Here's how the part is built. I have some questions about the finished solid (model axes, mm). A direction names the side the tool comes from. Coordinates: 2 decimals unless noted, no trailing zeros. Write each loop counter-clockwise with the first axis right and the second up, starting at its lowest first coordinate (ties: lowest second). Pieces come first, ordered by that corner, then holes. Notation, with made-up numbers: (49, -24) -> (83, -24) arc R8 cw to (83, -9) -> close; hole circle Ø5 at (-0.5, 25). An arc over 180 degrees is marked (long way). Use a Markdown table: item, result. Add a question column.
Item 1: If we mould it in two halves opening along Z, with no side actions, what happens to faces 6 (the flat face through (-2.2, 23, 0)), 7 (the flat face through (0, -34.6, 0)), 8 (the flat face through (-2.2, -2, 0)), 9 (the cylindrical face through (1.08, 9.86, 4.88))? For each: pulls with the +Z half, pulls with the -Z half, needs draft (parallel to the pull), parting line crosses it, or undercut.
Item 2: On a 3-axis mill with a long thin cutter (end or side, diameter ignored), from which of +Z, -Z, +X, -X, +Y, -Y can I reach the whole of each face in a straight line? I mean faces 1 (the flat face through (0, 91, 0)), 2 (the cylindrical face through (3.695, -17.058, 1.532)), 3 (the flat face through (-3, 20, 0)), 4 (the cylindrical face through (3.695, 55.003, -1.532)), 5 (the flat face through (-2.2, 72, 0)). Say none if no direction works.
Item 3: Imagine slicing it at D-D, the plane y = 6. Write out the boundary of the cut face in (x, z), and give its area (3 significant figures).
Item 4: Will these pins go through, and if not, where does the flat tip stop? pin 1 Ø0.8 at (x, y) = (-3, -3.5) entering from -Z; pin 2 Ø1.7 at (x, y) = (-3, 71.5) entering from -Z; pin 3 Ø1.7 at (x, y) = (-2.5, 71) entering from +Z.
Item 5: If I drill on line 1 along Y through (x, z) = (-3.5, 2); line 2 along X through (y, z) = (-24, -0.25); line 3 along Z through (x, y) = (3, 6.5), over which ranges is the centre line in solid material (lowest first)? Write a range as from..to.
Item 6: Imagine slicing it at B-B, the plane y = -18. Write out the boundary of the cut face in (x, z), and give its area (3 significant figures).
Item 7: Imagine slicing it at C-C, the plane y = 23. Write out the boundary of the cut face in (x, z).
Item 8: Imagine slicing it at A-A, the plane x = 0. Write out the boundary of the cut face in (y, z), and give its area (3 significant figures).
Autodesk Inventor part; units mm, degrees
ref_plane "作業平面1" through (0, -34.6, 4) normal (0, 0, 1) x (1, 0, 0)
ref_plane "作業平面2" through (-4, 0, 0) normal (-1, 0, 0) x (0, -1, 0)
ref_plane "YZ Plane" through (0, 0, 0) normal (1, 0, 0) x (0, 1, 0)
sketch "スケッチ1" plane through (0, 0, 0) normal (0, 1, 0) x (-1, 0, 0)
  circle A0 centre (0, 0) radius 5
  dimension "d0" = 10
extrude "押し出し1" add sketch "スケッチ1" along normal blind 20
sketch "スケッチ2" plane through (0, 20, 0) normal (0, 1, 0) x (1, 0, 0)
  circle A0 centre (0, 0) radius 4
  dimension "d3" = 8
extrude "押し出し2" add sketch "スケッチ2" along normal blind 71
sketch "スケッチ3" plane through (0, 0, 0) normal (0, -1, 0) x (1, 0, 0)
  circle A0 centre (0, 0) radius 4
  dimension "d6" = 8
extrude "押し出し3" add sketch "スケッチ3" along normal blind 34.6
sketch "スケッチ4" plane through (0, -34.6, 0) normal (0, -1, 0) x (1, 0, 0)
  circle A0 centre (0, 0) radius 4
  point P0 (0, 4)
ref_plane "作業平面1" through (0, -34.6, 4) normal (0, 0, 1) x (1, 0, 0)
sketch "スケッチ7" plane through (0, -34.6, 4) normal (0, 0, 1) x (1, 0, 0)
  line L0 (-1.5, 5) -> (1.5, 5)
  line L1 (1.5, 5) -> (1.5, 21)
  line L2 (1.5, 21) -> (-1.5, 21)
  line L3 (-1.5, 21) -> (-1.5, 5)
  line L4 (-1.5, 5) -> (1.5, 21) construction
  line L5 (1.5, 5) -> (-1.5, 21) construction
  line L6 (-4, 0) -> (4, 0)
  line L7 (-1.5, 104.6) -> (1.5, 104.6)
  line L8 (1.5, 104.6) -> (1.5, 120.6)
  line L9 (1.5, 120.6) -> (-1.5, 120.6)
  line L10 (-1.5, 120.6) -> (-1.5, 104.6)
  line L11 (-1.5, 104.6) -> (1.5, 120.6) construction
  line L12 (1.5, 104.6) -> (-1.5, 120.6) construction
  line L13 (4, 125.6) -> (-4, 125.6)
  point P0 (0, 34.6)
  point P1 (0, 13)
  point P2 (0, 112.6)
  dimension "d17" = 3
  dimension "d18" = 16
  dimension "d19" = 5
  dimension "d20" = 3
  dimension "d21" = 16
  dimension "d22" = 5
extrude "押し出し5" [suppressed]
sketch "スケッチ8" plane through (0, 20, 0) normal (0, 1, 0) x (1, 0, 0)
  circle A0 centre (0, 0) radius 5
  dimension "d25" = 10
extrude "押し出し6" [suppressed]
sketch "スケッチ9" plane through (0, 0, 0) normal (0, -1, 0) x (1, 0, 0)
  circle A0 centre (0, 0) radius 5
  circle A1 centre (0, 0) radius 5
  dimension "d28" = 10
extrude "押し出し7" [suppressed]
sketch "スケッチ10" plane through (0, 0, 0) normal (0, -1, 0) x (1, 0, 0)
  circle A0 centre (0, 0) radius 4
  point P0 (-4, 0)
ref_plane "作業平面2" through (-4, 0, 0) normal (-1, 0, 0) x (0, -1, 0)
sketch "スケッチ11" plane through (-4, 0, 0) normal (-1, 0, 0) x (0, -1, 0)
  line L0 (0, -1.5) -> (5, -1.5)
  line L1 (5, -1.5) -> (5, 1.5)
  line L2 (5, 1.5) -> (0, 1.5)
  line L3 (0, 1.5) -> (0, -1.5)
  line L4 (0, -1.5) -> (5, 1.5) construction
  line L5 (5, -1.5) -> (0, 1.5) construction
  line L6 (0, 5) -> (0, -5)
  line L7 (-25, 1.5) -> (-20, 1.5)
  line L8 (-20, 1.5) -> (-20, -1.5)
  line L9 (-20, -1.5) -> (-25, -1.5)
  line L10 (-25, -1.5) -> (-25, 1.5)
  line L11 (-25, 1.5) -> (-20, -1.5) construction
  line L12 (-20, 1.5) -> (-25, -1.5) construction
  line L13 (-20, 5) -> (-20, -5)
  line L14 (-80, 1.5) -> (-64, 1.5)
  line L15 (-64, 1.5) -> (-64, -1.5)
  line L16 (-64, -1.5) -> (-80, -1.5)
  line L17 (-80, -1.5) -> (-80, 1.5)
  line L18 (-80, 1.5) -> (-64, -1.5) construction
  line L19 (-64, 1.5) -> (-80, -1.5) construction
  line L20 (-91, 4) -> (-91, -4)
  point P0 (0, 0)
  point P1 (2.5, 0)
  point P2 (-22.5, 0)
  point P3 (-72, 0)
  dimension "d31" = 5
  dimension "d32" = 3
  dimension "d33" = 0
  dimension "d34" = 5
  dimension "d35" = 3
  dimension "d36" = 0
  dimension "d39" = 16
  dimension "d40" = 3
  dimension "d41" = 11
extrude "押し出し8" cut sketch "スケッチ11" against normal blind 1.8
properties part number "shoulder2_shaft" material "鋼、炭素鋼"
Ans:
| question | item | result |
|---|---|---|
| 1 | face 6 | undercut |
| 1 | face 7 | needs draft |
| 1 | face 8 | undercut |
| 1 | face 9 | parting line crosses it |
| 2 | face 1 | +Z, -Z, +X, -X, +Y |
| 2 | face 2 | -Y |
| 2 | face 3 | none |
| 2 | face 4 | +Y |
| 2 | face 5 | -X |
| 3 | outline | circle Ø10 at (0, 0) |
| 3 | area | 78.5 mm^2 |
| 4 | pin 1 | stops at z = -3.04 |
| 4 | pin 2 | stops at z = -3.37 |
| 4 | pin 3 | stops at z = 3.64 |
| 5 | line 1 | y = 0..20 |
| 5 | line 2 | x = -3.99..3.99 |
| 5 | line 3 | z = -4..4 |
| 6 | outline | circle Ø8 at (0, 0) |
| 6 | area | 50.3 mm^2 |
| 7 | outline | (-3.71, -1.5) arc R4 ccw (long way) to (-3.71, 1.5) -> (-2.2, 1.5) -> (-2.2, -1.5) -> close |
| 8 | outline | (-34.6, -4) -> (0, -4) -> (0, -5) -> (20, -5) -> (20, -4) -> (91, -4) -> (91, 4) -> (20, 4) -> (20, 5) -> (0, 5) -> (0, 4) -> (-34.6, 4) -> close |
| 8 | area | 1,040 mm^2 |
